Geometry: final body of the model. Coordinates: model frame, mm. Face numbers are marked on the shaded views. Give positions to 0.01 mm unless a question says otherwise; leave off trailing zeros. Write each loop counter-clockwise with the first axis right and the second up, starting at its lowest first coordinate (ties: lowest second). Pieces come first, ordered by that corner, then holes. Notation, with made-up numbers: (2.25, 62) - (36.25, 62) arc R13 cw to (36.25, 74) - close; hole circle Ø1 at (-2, 26.25). An arc over 180 degrees is marked (long way). Use CSV: the item, a comma, the result in double quotes. Start each with the question number.
(1) Section C-C on y = -8.75. Output: boundary loops of the cut face in (x, z), and give its area (3 significant figures).
(2) Section D-D on x = 12. Output: boundary loops of the cut face in (y, z).
(3) Line query: probe 1 along X at (y, z) = (-2.25, 4); probe 2 along X at (y, z) = (2.5, -4.5); probe 3 along Z at (x, y) = (-8.5, -0.25). Output: solid intervals per line, ascending. Write a range as [from, to].
(4) Draft query along Z for the marked faces 1 and 2. Return one class per face: released by +Z, released by -Z, zero draft, split by the parting line, or undercut.
(5) Section B-B on x = -14.5. Output: boundary loops of the cut face in (y, z), and give its area (3 significant figures).
(6) Section A-A on z = 0. Output: boundary loops of the cut face in (x, y).
(7) First-contact query: pin 1 Ø1 at (x, z) = (5.5, -4.5) entering from -Y; pin 2 Ø2 at (x, y) = (9, 1.5) entering from -Z; pin 3 Ø1.5 at (x, y) = (13.5, 3) entering from -Z. Flat tips, straight axial feed; report the tip coordinate or a pass-through.
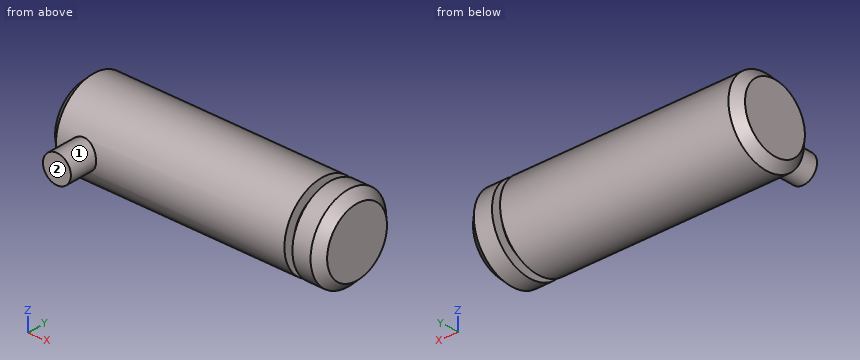
from build123d import *

# Parameters (mm, degrees)
SKETCH1_W           = 34
SKETCH1_H           = 6
SKETCH3_R           = 2
BOSS_EXTRUDE1_DEPTH = 10
SKETCH4_W           = 5
SKETCH4_H           = 6
SKETCH5_W           = 1.15
SKETCH5_H           = 1.5


with BuildPart() as part:
    # Sketch1 → Revolve1 (revolve)
    with BuildSketch(Plane.XY):
        with Locations((-2.5, 3)):
            Rectangle(SKETCH1_W, SKETCH1_H)
    revolve(axis=Axis((14.5, 0, 0), (-1, 0, 0)))

    # Sketch2 → Cut-Revolve1 (revolve, cut)
    with BuildSketch(Plane.XY):
        Polygon((-19.5, 4.75), (-18.25, 6), (-19.5, 6), align=None)
    revolve(axis=Axis((29, 0, 0), (-1, 0, 0)), mode=Mode.SUBTRACT)

    # Sketch3 → Boss-Extrude1 (add)
    with BuildSketch(Plane(origin=(0, 0, 0), x_dir=(1, 0, 0), z_dir=(0, 1, 0))):
        with Locations((-14.5, 0)):
            Circle(SKETCH3_R)
    extrude(amount=-BOSS_EXTRUDE1_DEPTH)

    # Sketch4 → Revolve2 (revolve)
    with BuildSketch(Plane.XY):
        with Locations((17, 3)):
            Rectangle(SKETCH4_W, SKETCH4_H)
    revolve(axis=Axis((19.5, 0, 0), (-1, 0, 0)))

    # Sketch5 → Cut-Revolve2 (revolve, cut)
    with BuildSketch(Plane.XY):
        with Locations((15.075, 5.25)):
            Rectangle(SKETCH5_W, SKETCH5_H)
    revolve(axis=Axis((29, 0, 0), (-1, 0, 0)), mode=Mode.SUBTRACT)

    # Sketch6 → Cut-Revolve3 (revolve, cut)
    with BuildSketch(Plane.XY):
        Polygon((18.25, 6), (19.5, 4.75), (19.5, 6), align=None)
    revolve(axis=Axis((29, 0, 0), (-1, 0, 0)), mode=Mode.SUBTRACT)


solid = part.part
Check values:
1,outline,"circle Ø4 at (-14.5, 0)"
1,area,"12.6 mm²"
2,outline,"circle Ø12 at (0, 0)"
3,probe 1,"x = [-19.5, 14.5], [15.65, 19.5]"
3,probe 2,"x = [-19.1, 14.5], [15.65, 19.1]"
3,probe 3,"z = [-5.99, 5.99]"
4,face 1,"split by the parting line"
4,face 2,"zero draft"
5,outline,"(-10, -2) - (-5.66, -2) arc R6 ccw (long way) to (-5.66, 2) - (-10, 2) - close"
5,area,"130 mm²"
6,outline,"(-19.5, -4.75) - (-18.25, -6) - (-16.5, -6) - (-16.5, -10) - (-12.5, -10) - (-12.5, -6) - (14.5, -6) - (14.5, -4.5) - (15.65, -4.5) - (15.65, -6) - (18.25, -6) - (19.5, -4.75) - (19.5, 4.75) - (18.25, 6) - (15.65, 6) - (15.65, 4.5) - (14.5, 4.5) - (14.5, 6) - (-18.25, 6) - (-19.5, 4.75) - close"
7,pin 1,"stops at y = -4.47"
7,pin 2,"stops at z = -5.98"
7,pin 3,"stops at z = -5.56"
